Input: part model. Units: mm. Frame: model coordinates. A direction names the side the tool comes from. Give positions to 0.01 mm unless a question says otherwise; leave off trailing zeros. Loops run counter-clockwise (first coordinate to the right, second up) from the corner with the lowest first, then second, coordinate; pieces in that order, holes last. Notation, with made-up numbers: (-35.75, 70.25) - (-17.75, 70.25) arc R29 ccw to (-17.75, 90.25) - close; hole circle Ø3 at (64, 72). An arc over 180 degrees is marked (long way). Answer as a JSON object with one key per item and string values.
from build123d import *

# Parameters (mm, degrees)
F1_DEPTH = 2.5
F2_W     = 2.3
F2_H     = 9.6
F3_DEPTH = 3.4
F5_DEPTH = 10


# Not quite as in the source:
# - ends of sketch curves that miss each other by under 0.0002 mm in the source are joined
# - the dataset's text gives a spline's control points without its knots; the knots are read off the source's solid


with BuildPart() as f1:
    # F0 (on Top) → F1 (new body)
    with BuildSketch(Plane.XY):
        with BuildLine():
            Line((32.5, -4.8), (32.5, 0))
            Line((32.5, 0), (32.5, 4.8))
            Line((32.5, 4.8), (22.5, 4.8))
            Line((22.5, 4.8), (22.5, 7.5))
            Line((22.5, 7.5), (18.5, 7.5))
            add(Edge.make_bspline(
                [(18.5, 7.5), (16.6328875571, 8.7478424674), (12.4879926615, 11.0335251601), (7.8863773573, 13.5145464122), (2.5994103613, 13.8122400643), (0, 13.9694881193)],
                knots=[0, 0, 0, 0, 0.3363717727, 0.6336483956, 0.9777931055, 0.9777931055, 0.9777931055, 0.9777931055], degree=3))
            add(Edge.make_bspline(
                [(-18.5, 7.5), (-16.6328875571, 8.7478424674), (-12.4879926615, 11.0335251601), (-7.8863773573, 13.5145464122), (-2.5994103613, 13.8122400643), (0, 13.9694881193)],
                knots=[0, 0, 0, 0, 0.3363717727, 0.6336483956, 0.9777931055, 0.9777931055, 0.9777931055, 0.9777931055], degree=3))
            Line((-18.5, 7.5), (-22.5, 7.5))
            Line((-22.5, 7.5), (-22.5, 4.8))
            Line((-22.5, 4.8), (-32.5, 4.8))
            Line((-32.5, 4.8), (-32.5, 0))
            Line((-32.5, 0), (-32.5, -4.8))
            Line((-32.5, -4.8), (-22.5, -4.8))
            Line((-22.5, -4.8), (-22.5, -7.5))
            Line((-22.5, -7.5), (-18.5, -7.5))
            add(Edge.make_bspline(
                [(-18.5, -7.5), (-16.6328875571, -8.7478424674), (-12.4879926615, -11.0335251601), (-7.8863773573, -13.5145464122), (-2.5994103613, -13.8122400643), (0, -13.9694881193)],
                knots=[0, 0, 0, 0, 0.3363717727, 0.6336483956, 0.9777931055, 0.9777931055, 0.9777931055, 0.9777931055], degree=3))
            add(Edge.make_bspline(
                [(18.5, -7.5), (16.6328875571, -8.7478424674), (12.4879926615, -11.0335251601), (7.8863773573, -13.5145464122), (2.5994103613, -13.8122400643), (0, -13.9694881193)],
                knots=[0, 0, 0, 0, 0.3363717727, 0.6336483956, 0.9777931055, 0.9777931055, 0.9777931055, 0.9777931055], degree=3))
            Line((18.5, -7.5), (22.5, -7.5))
            Line((22.5, -7.5), (22.5, -4.8))
            Line((22.5, -4.8), (32.5, -4.8))
        make_face()
        with BuildLine():
            Line((-18.5, 0), (-18.5, 5.9768469073))
            Line((-18.5, 5.9768469073), (-17.4557828979, 6.6914400202))
            add(Edge.make_bspline(
                [(-17.4557828979, 6.6914400202), (-16.8874977541, 7.0617589277), (-15.5631242254, 7.8773690533), (-13.8072733089, 8.8734333253), (-12.5364597536, 9.5720832259), (-11.8350717008, 9.9552778211), (-11.1621909622, 10.3213808687), (-10.364996594, 10.7418634519), (-9.4382542316, 11.1823324733), (-8.4958782817, 11.5579825068), (-7.6562822144, 11.8178001131), (-6.921672188, 11.9930107338), (-6.1338774618, 12.1498095188), (-5.0696801932, 12.3116557143), (-3.7025355233, 12.4602871457), (-2.0018671704, 12.5972327818), (-0.7534045854, 12.6716577772), (5.394e-07, 12.717197038)],
                knots=[0.0214889286, 0.0214889286, 0.0214889286, 0.0214889286, 0.125, 0.25, 0.3125, 0.34375, 0.375, 0.4375, 0.5, 0.5625, 0.625, 0.65625, 0.6875, 0.75, 0.8125, 0.875, 0.9744706617, 0.9744706617, 0.9744706617, 0.9744706617], degree=3))
            add(Edge.make_bspline(
                [(17.4557781808, 6.6914327816), (16.8874977541, 7.0617589277), (15.5631242254, 7.8773690533), (13.8072733089, 8.8734333253), (12.5364597536, 9.5720832259), (11.8350717008, 9.9552778211), (11.1621909622, 10.3213808687), (10.364996594, 10.7418634519), (9.4382542316, 11.1823324733), (8.4958782817, 11.5579825068), (7.6562822144, 11.8178001131), (6.921672188, 11.9930107338), (6.1338774618, 12.1498095188), (5.0696801932, 12.3116557143), (3.7025355233, 12.4602871457), (2.0018675288, 12.597232753), (0.7534053146, 12.6716577338), (5.394e-07, 12.717197038)],
                knots=[0.0214889286, 0.0214889286, 0.0214889286, 0.0214889286, 0.125, 0.25, 0.3125, 0.34375, 0.375, 0.4375, 0.5, 0.5625, 0.625, 0.65625, 0.6875, 0.75, 0.8125, 0.875, 0.9744706144, 0.9744706144, 0.9744706144, 0.9744706144], degree=3))
            Line((17.4557781808, 6.6914327816), (18.5, 5.9768469073))
            Line((18.5, 5.9768469073), (18.5, 5))
            Line((18.5, 5), (18.5, 0))
            Line((18.5, 0), (18.5, -5.9768469073))
            Line((18.5, -5.9768469073), (17.4557828979, -6.6914400202))
            add(Edge.make_bspline(
                [(17.4557828979, -6.6914400202), (16.8874977541, -7.0617589277), (15.5631242254, -7.8773690533), (13.8072733089, -8.8734333253), (12.5364597536, -9.5720832259), (11.8350717008, -9.9552778211), (11.1621909622, -10.3213808687), (10.364996594, -10.7418634519), (9.4382542316, -11.1823324733), (8.4958782817, -11.5579825068), (7.6562822144, -11.8178001131), (6.921672188, -11.9930107338), (6.1338774618, -12.1498095188), (5.0696801932, -12.3116557143), (3.7025355233, -12.4602871457), (2.0018673502, -12.5972327673), (0.7534049513, -12.6716577554), (0, -12.7171970054)],
                knots=[0.0214889286, 0.0214889286, 0.0214889286, 0.0214889286, 0.125, 0.25, 0.3125, 0.34375, 0.375, 0.4375, 0.5, 0.5625, 0.625, 0.65625, 0.6875, 0.75, 0.8125, 0.875, 0.974470638, 0.974470638, 0.974470638, 0.974470638], degree=3))
            add(Edge.make_bspline(
                [(-17.4557781808, -6.6914327816), (-16.8874977541, -7.0617589277), (-15.5631242254, -7.8773690533), (-13.8072733089, -8.8734333253), (-12.5364597536, -9.5720832259), (-11.8350717008, -9.9552778211), (-11.1621909622, -10.3213808687), (-10.364996594, -10.7418634519), (-9.4382542316, -11.1823324733), (-8.4958782817, -11.5579825068), (-7.6562822144, -11.8178001131), (-6.921672188, -11.9930107338), (-6.1338774618, -12.1498095188), (-5.0696801932, -12.3116557143), (-3.7025355233, -12.4602871457), (-2.0018673502, -12.5972327673), (-0.7534049513, -12.6716577554), (0, -12.7171970054)],
                knots=[0.0214889286, 0.0214889286, 0.0214889286, 0.0214889286, 0.125, 0.25, 0.3125, 0.34375, 0.375, 0.4375, 0.5, 0.5625, 0.625, 0.65625, 0.6875, 0.75, 0.8125, 0.875, 0.974470638, 0.974470638, 0.974470638, 0.974470638], degree=3))
            Line((-17.4557781808, -6.6914327816), (-18.5, -5.9768469073))
            Line((-18.5, -5.9768469073), (-18.5, 0))
        make_face(mode=Mode.SUBTRACT)
    extrude(amount=-F1_DEPTH)

    # F2 (on face) → F3 (join)
    with BuildSketch(Plane.XY):
        with Locations((19.65, 0)):
            Rectangle(F2_W, F2_H)
        with Locations((-19.65, 0)):
            Rectangle(F2_W, F2_H)
    extrude(amount=F3_DEPTH)

    # F4 (on face) → F5 (join)
    with BuildSketch(Plane.XZ.offset(4.8)):
        Polygon((18.5, 5.9), (18.5, 3.4), (22.5, 3.4), (20.5, 5.9), align=None)
        Polygon((-20.5, 5.9), (-22.5, 3.4), (-18.5, 3.4), (-18.5, 5.9), align=None)
    extrude(amount=-F5_DEPTH)


solid = f1.part
Item 1: Mould query, pull axis X, two halves, no side actions, for faces 1 (the face through (-20, 4.8, 2)), 2 (the face through (18.5, 0, 2)), 3 (the face through (22.5, -6, -1)). Classes: released by +X, released by -X, zero draft, split by the parting line, or undercut.
Geometry check:
{"face 1": "zero draft", "face 2": "undercut", "face 3": "released by +X"}
Item 2: Cut plane B-B (z = 2). Return loops of the section in (x, y).
Geometry check:
{"outline": "(-20.8, -4.8) - (-18.5, -4.8) - (-18.5, 4.8) - (-20.8, 4.8) - close; (18.5, -4.8) - (20.8, -4.8) - (20.8, 4.8) - (18.5, 4.8) - close"}
Item 3: Access query for faces 4 (the face through (-20.8, 0, 2)), 5 (the face through (20, -4.8, 3)), 6 (the face through (20, 4.8, 2)), 7 (the face through (20.8, 0, 2)), 8 (the face through (21, 7.5, -1)). Directions: +Z, -Z, +X, -X, +Y, -Y. A direction counts if a zero-diameter tool reaches every point of the face in a straight line with its end or side. Return the directions, or none.
Geometry check:
{"face 4": "-X, +Y, -Y", "face 5": "+Z, +X, -X, -Y", "face 6": "+X, -X, +Y", "face 7": "+X, +Y, -Y", "face 8": "+Z, -Z, +X, +Y"}
Item 4: Contact query for flat-ended pins moving along their axis: P1, Ø1.7, axis at y = -2, z = 2.5, coming from the +X side; P2, Ø1.2, axis at x = 20, z = -1, coming from the -Y side; P3, Ø3, axis at x = 20.5, z = 4, coming from the -Y side. Output: stop coordinate, or through.
Geometry check:
{"P1": "stops at x = 20.8", "P2": "stops at y = -7.5", "P3": "stops at y = -4.8"}
Item 5: Cut plane C-C (x = 26). Return loops of the section in (y, z), then the cut area to 3 significant figures.
Geometry check:
{"outline": "(-4.8, -2.5) - (4.8, -2.5) - (4.8, 0) - (-4.8, 0) - close", "area": "24.0 mm2"}
Item 6: Material intervals for line 1 (X direction, y = -1.5, z = -1.75); line 2 (X direction, y = 2, z = 1.25); line 3 (Y direction, x = -18, z = -0.25), sorted ascending. Write a range as [from, to].
Geometry check:
{"line 1": "x = [-32.5, -18.5], [18.5, 32.5]", "line 2": "x = [-20.8, -18.5], [18.5, 20.8]", "line 3": "y = [-7.83, -6.32], [6.32, 7.83]"}
Item 7: Cut plane A-A (y = -1.5). Return loops of the section in (x, z).
Geometry check:
{"outline": "(-32.5, -2.5) - (-18.5, -2.5) - (-18.5, 5.9) - (-20.5, 5.9) - (-22.5, 3.4) - (-20.8, 3.4) - (-20.8, 0) - (-32.5, 0) - close; (18.5, -2.5) - (32.5, -2.5) - (32.5, 0) - (20.8, 0) - (20.8, 3.4) - (22.5, 3.4) - (20.5, 5.9) - (18.5, 5.9) - close"}
